For this review, use the dimensioned drawing (mm, ordinates from the lowest corner) and the shaded views. A direction names the side the tool comes from. Round coordinates to 2 decimals unless told otherwise and drop trailing zeros. Write each loop counter-clockwise with the first axis right and the second up, starting at its lowest first coordinate (ties: lowest second). Pieces come first, ordered by that corner, then holes. Notation, with made-up numbers: (-23, 32.5) -> (1, 32.5) arc R20 cw to (1, 63.5) -> close; hole circle Ø4 at (8, -28). An arc over 180 degrees is marked (long way). Write each question's results on one line, items separated by ' | '. Start each with the question number.
Item 1: Add section D-D (z = 6). State the section outline as (x, y) points.
Item 2: Clearance check with flat-ended pins moving along their axes: pin 1 (0.6 mm diameter, centred on x = 5, y = 5.5, fed in from -Z); pin 2 (5 mm diameter, centred on x = 12.5, y = 14, fed in from -Z); pin 3 (1.5 mm diameter, centred on y = 11.5, z = 14.5, fed in from -X). State where each tip first meets the part, or that it passes through.
Item 3: To check wall thickness, follow line 1 along Z through (x, y) = (10, 14.5); line 2 along X through (y, z) = (15.5, 26.5); line 3 along X through (y, z) = (14.5, 16). State the ranges of each line that lie inside material, in increasing order.
Item 4: Add section C-C (z = 13.5). State the section outline as (x, y) points, plus the area to 3 significant figures.
Item 5: Tool access review of the marked faces 1 and 2: name each direction out of +Z, -Z, +X, -X, +Y, -Y from which nothing blocks a thin tool from reaching the whole face with its end or side.
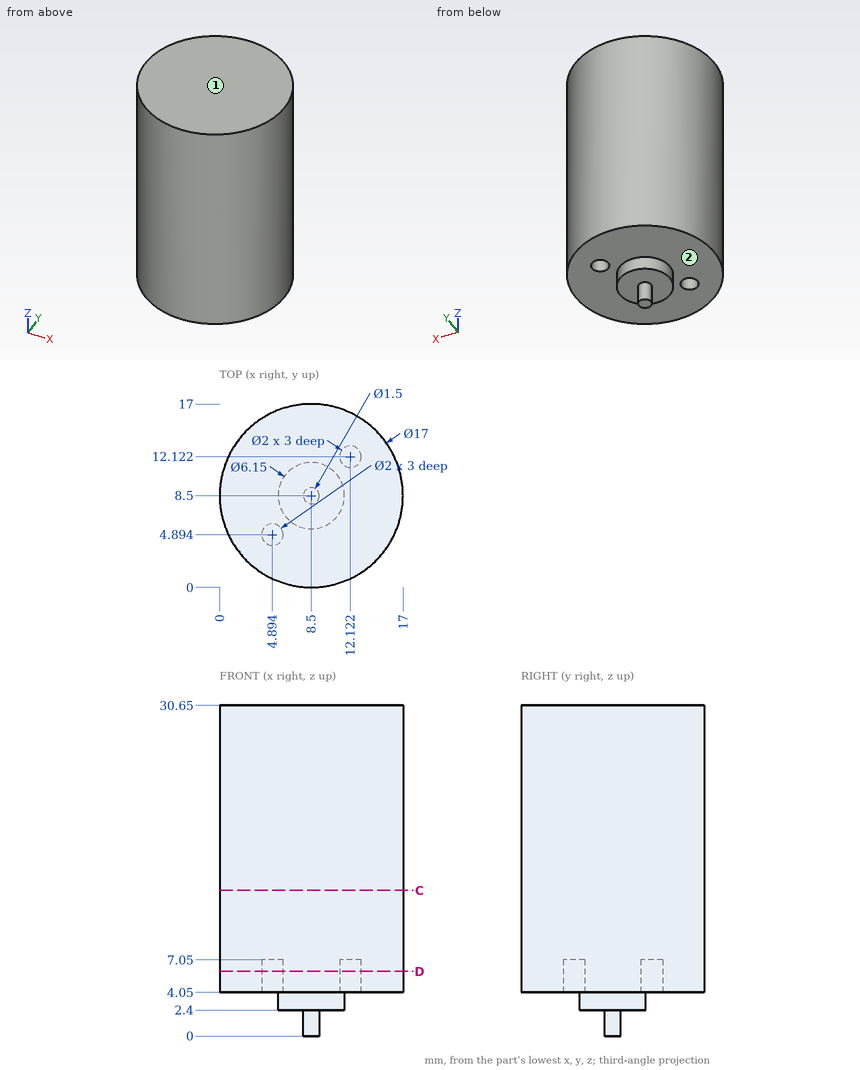
Responses:
1) outline: circle Ø17 at (8.5, 8.5); hole circle Ø2 at (4.89, 4.89); hole circle Ø2 at (12.12, 12.12)
2) pin 1: stops at z = 7.05 | pin 2: stops at z = 4.05 | pin 3: stops at x = 0.3
3) line 1: z = 4.05 to 30.65 | line 2: x = 3.68 to 13.32 | line 3: x = 2.48 to 14.52
4) outline: circle Ø17 at (8.5, 8.5) | area: 227 mm^2
5) face 1: +Z, +X, -X, +Y, -Y | face 2: -Z
